Check sheet for the modelled part. Datum: model origin and axes. Units: mm. Face numbers are marked on the shaded views. A direction names the side the tool comes from. Round coordinates to 2 decimals unless told otherwise and drop trailing zeros. Order: outer loops, then holes, each group sorted by start corner. A loop starts at its lowest first (then second) coordinate and runs counter-clockwise, first axis right, second up. Notation, with made-up numbers: (-39, 8.5) -> (-14, 8.5) arc R16 cw to (-14, 32.5) -> close; hole circle Ø8 at (54.25, -10.75). An arc over 180 degrees is marked (long way). Answer in a Markdown table with one row per item. Add a question column.
1. Access from +Z, -Z, +X, -X, +Y, -Y to the whole of each face (thin tool, end or side, straight path). Record for the marked faces 1 and 2.
2. Depth check by flat-ended pin: P1, Ø4, axis at x = -276.5, y = -38.5, coming from the -Z side; P2, Ø6, axis at x = -201, y = -89.5, coming from the +Z side; P3, Ø3.5, axis at x = -220.5, z = 2, coming from the +Y side; P4, Ø2.5, axis at x = -78, z = 1, coming from the -Y side. Enter the tip coordinate at first touch or a pass-through.
3. Sectioned sample at D-D, the plane x = -153.5. Record the boundary of the cut face in (y, z), then the cut area to 3 significant figures.
4. Sectioned sample at C-C, the plane z = -73. Record the boundary of the cut face in (x, y).
5. Sectioned sample at B-B, the plane x = -368. Record the boundary of the cut face in (y, z), then the cut area to 3 significant figures.
6. Material ranges on L1, parallel to Y at x = -222, z = -69; L2, parallel to Z at x = -211.5, y = -14; L3, parallel to Z at x = -207.5, y = -4.5, recorded low to high. Write a range as from..to.
7. Sectioned sample at A-A, the plane y = -48. Record the boundary of the cut face in (x, z).
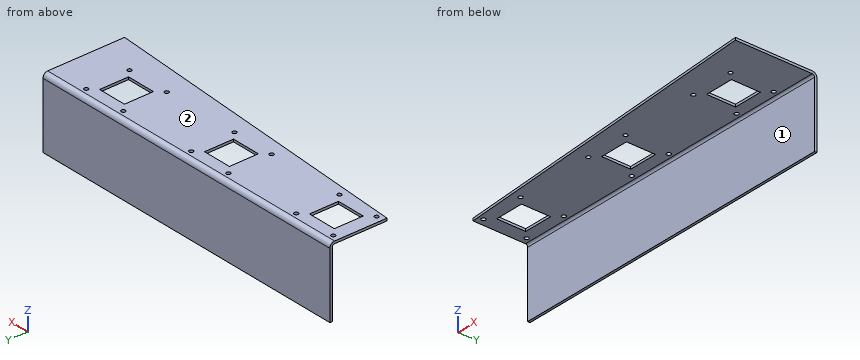
Autodesk Inventor part; units mm, degrees
ref_plane "YZ Plane" through (0, 0, 0) normal (1, 0, 0) x (0, 1, 0)
ref_plane "XZ Plane" through (0, 0, 0) normal (0, 1, 0) x (-1, 0, 0)
ref_plane "XY Plane" through (0, 0, 0) normal (0, 0, 1) x (1, 0, 0)
sketch "Sketch1" plane through (0, 0, 0) normal (0, 0, 1) x (1, 0, 0)
  line L0 (0, 0) -> (-410, 0)
  line L1 (0, -100) -> (0, 0)
  line L2 (-410, 0) -> (-410, -70)
  line L3 (-410, -70) -> (0, -100)
  point P0 (0, -50)
  dimension "d32" = 100
  dimension "d60" = 70
  dimension "d61" = 410
extrude "Plate1" add sketch "Sketch1" along normal blind 3
sketch "Sketch8" plane through (0, 0, 3) normal (0, 0, 1) x (1, 0, 0)
  line L0 (-57.25, -55.75) -> (-92.75, -55.75)
  line L1 (-92.75, -55.75) -> (-92.75, -20.25)
  line L2 (-92.75, -20.25) -> (-57.25, -20.25)
  line L3 (-57.25, -20.25) -> (-57.25, -55.75)
  line L4 (-57.25, -55.75) -> (-92.75, -20.25) construction
  line L5 (-92.75, -55.75) -> (-57.25, -20.25) construction
  circle A0 centre (-48.4835, -64.5165) radius 2.5
  circle A1 centre (-101.5165, -64.5165) radius 2.5
  circle A2 centre (-101.5165, -11.4835) radius 2.5
  circle A3 centre (-48.4835, -11.4835) radius 2.5
  circle A4 centre (-75, -38) radius 37.5 construction
  line L6 (0, 0) -> (0, -100)
  line L7 (-410, 0) -> (0, 0)
  line L8 (-92.75, -55.75) -> (-101.5165, -64.5165) construction
  dimension "d51" = 35.5
  dimension "d52" = 35.5
  dimension "d53" = 5
  dimension "d72" = 75
  dimension "d73" = 38
  dimension "d74" = 12.3977
  dimension "d75" = 75
extrude "Cut3" cut sketch "Sketch8" against normal blind 3
pattern_linear "Rectangular Pattern1" count 3 spacing 150 along (-1, 0, 0) of "Cut3"
sketch "Sketch9" plane through (0, -3, 3) normal (0, 1, 0) x (-1, 0, 0)
  line L0 (410, 0) -> (0, 0)
  line L1 (0, 0) -> (0, -86)
  line L2 (0, -86) -> (410, -86)
  line L3 (410, -86) -> (410, 0)
edge flange "Flange3" height 86 angle 90 thickness 3 bend radius 2.75 thickness toward (0, 1, 0) relief round relief width 3 relief depth 1.5 edges at (-205, 0, 0) wall of the first edge with corners at (-410, -3, 3) (0, -3, 3) (0, -3, -83) (-410, -3, -83)
bend "Bend3"
corner "Corner3"
equation "\"d32\" = Main_way_hight"
equation "\"d61\" = Main_way_lenth"
equation "\"d51\" = d52"
equation "\"d55\" = Thickness"
equation "\"d2\" = Thickness"
equation "\"d62\" = BendReliefWidth"
equation "\"d63\" = BendReliefDepth"
equation "\"d64\" = MinimumRemnant"
equation "\"d65\" = TransitionRadius"
equation "\"d66\" = MAIN_7_central_window_width + 2 * Thickness"
equation "\"d68\" = BendRadius"
equation "\"d69\" = CornerReliefSize"
equation "\"d70\" = GapSize"
equation "\"d71\" = JacobiRadiusSize"
equation "\"BendReliefWidth\" = Thickness"
equation "\"BendReliefDepth\" = 0.5 * Thickness"
equation "\"CornerReliefSize\" = 4 * Thickness"
equation "\"MinimumRemnant\" = 2 * Thickness"
equation "\"TransitionRadius\" = BendRadius"
equation "\"JacobiRadiusSize\" = BendRadius"
equation "\"GapSize\" = Thickness"
equation "\"Main_way_hight\" = 100"
equation "\"Main_way_lenth\" = 410"
properties part number "ANP 1422 BOTTOM FDS diameter way up" material "Stainless Steel"
Answer key:
| question | item | result |
|---|---|---|
| 1 | face 1 | -Z, +X, -X, -Y |
| 1 | face 2 | +Z, +X, -X, +Y, -Y |
| 2 | P1 | stops at z = 0 |
| 2 | P2 | passes through |
| 2 | P3 | stops at y = -0.84 |
| 2 | P4 | stops at y = -94.38 |
| 3 | outline | (-88.77, 0) -> (-5.75, 0) arc R2.75 cw to (-3, -2.75) -> (-3, -83) -> (0, -83) -> (0, -2.75) arc R5.75 ccw to (-5.75, 3) -> (-88.77, 3) -> close |
| 3 | area | 510 mm² |
| 4 | outline | (-410, -3) -> (0, -3) -> (0, 0) -> (-410, 0) -> close |
| 5 | outline | (-73.07, 0) -> (-55.75, 0) -> (-55.75, 3) -> (-73.07, 3) -> close; (-20.25, 0) -> (-5.75, 0) arc R2.75 cw to (-3, -2.75) -> (-3, -83) -> (0, -83) -> (0, -2.75) arc R5.75 ccw to (-5.75, 3) -> (-20.25, 3) -> close |
| 5 | area | 356 mm² |
| 6 | L1 | y = -3..0 |
| 6 | L2 | z = 0..3 |
| 6 | L3 | z = -0.3..2.86 |
| 7 | outline | (-410, 0) -> (-392.75, 0) -> (-392.75, 3) -> (-410, 3) -> close; (-357.25, 0) -> (-242.75, 0) -> (-242.75, 3) -> (-357.25, 3) -> close; (-207.25, 0) -> (-92.75, 0) -> (-92.75, 3) -> (-207.25, 3) -> close; (-57.25, 0) -> (0, 0) -> (0, 3) -> (-57.25, 3) -> close |
